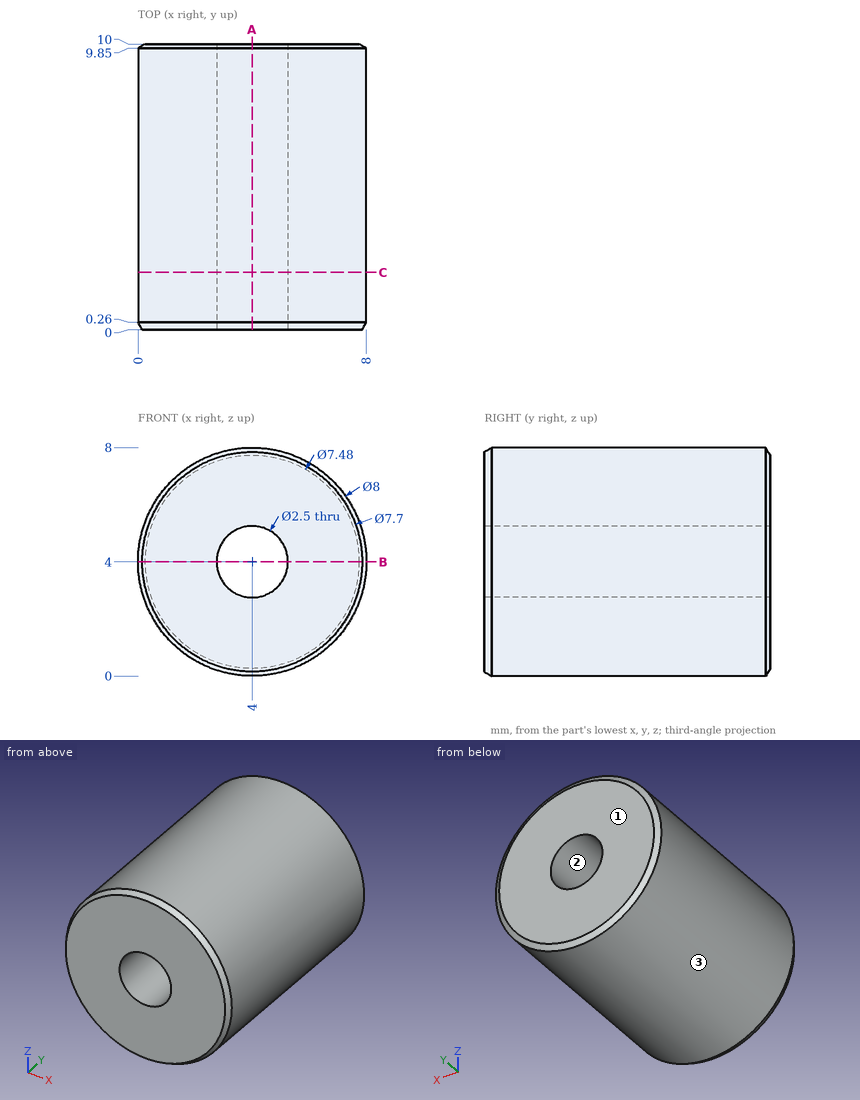
Can you work these out from the drawing? Everything is in mm from the part's minimum corner. Give positions to 0.01 mm unless a question says otherwise; leave off trailing zeros. Order: outer loops, then holes, each group sorted by start corner. A loop starts at its lowest first (then second) coordinate and runs counter-clockwise, first axis right, second up. Notation, with made-up numbers: M 83.5,78.5 L 96.5,78.5 A17 cw 96.5,107.5 Z; hole C 11,23 d3. An arc over 180 degrees is marked long. One line per question, with ' | ' between items.
1. We'd pull the mould along X, two halves only. Please class the marked faces 1, 2 and 3: +X half, -X half, draft (parallel to the pull), parting line (faces both ways), or undercut.
Results:
face 1: draft | face 2: undercut | face 3: parting line
2. I want a section at A-A (x = 4). List the corners of the cut face in (y, z) for me.
Results:
outline: M 0,0.15 L 0.26,0 L 9.85,0 L 10,0.26 L 10,2.75 L 0,2.75 Z; M 0,5.25 L 10,5.25 L 10,7.74 L 9.85,8 L 0.26,8 L 0,7.85 Z
3. I'm going to push a flat-ended pin straight in: pin 1 (2 mm diameter, centred on x = 6.5, y = 1.5, fed in from +Z). Where does the tip first touch, or does it pass through?
Results:
pin 1: z = 7.71
4. I want a section at C-C (y = 2). List the corners of the cut face in (x, z) for me.
Results:
outline: C 4,4 d8; hole C 4,4 d2.5
5. If I drill on line 1 (Z direction, x = 4, y = 3.25); line 2 (X direction, y = 5, z = 6.5), over which ranges is the centre line in solid material (lowest first)?
Results:
line 1: 0 to 2.75, 5.25 to 8 | line 2: 0.88 to 7.12
6. I want a section at B-B (z = 4). List the corners of the cut face in (x, y) for me.
Results:
outline: M 0,0.26 L 0.15,0 L 2.75,0 L 2.75,10 L 0.26,10 L 0,9.85 Z; M 5.25,0 L 7.85,0 L 8,0.26 L 8,9.85 L 7.74,10 L 5.25,10 Z
